Build history of the part. All positions in model axes, mm. A direction names the side the tool comes from. Round coordinates to 2 decimals unless told otherwise and drop trailing zeros. Write each loop counter-clockwise with the first axis right and the second up, starting at its lowest first coordinate (ties: lowest second). Pieces come first, ordered by that corner, then holes. Notation, with made-up numbers: M 3.25,59.5 L 32.25,59.5 A23 ccw 32.25,98.5 Z; hole C 50.5,-34 d6. An arc over 180 degrees is marked long. Write item = value, one per line.
from build123d import *

# Parameters (mm, degrees)
SKETCH1_W           = 60.96
SKETCH1_H           = 38.1
BOSS_EXTRUDE1_DEPTH = 104.775
SKETCH3_R           = 6.732897925
BOSS_EXTRUDE2_DEPTH = 20.0025
SKETCH2_R           = 6.865425502
BOSS_EXTRUDE3_DEPTH = 20.0025


with BuildPart() as part:
    # Sketch1 → Boss-Extrude1 (new body)
    with BuildSketch(Plane(origin=(0, 0, 0), x_dir=(0, 0, -1), z_dir=(1, 0, 0))):
        with Locations((30.48, 19.05)):
            Rectangle(SKETCH1_W, SKETCH1_H)
    extrude(amount=BOSS_EXTRUDE1_DEPTH)

    # Sketch3 → Boss-Extrude2 (add)
    with BuildSketch(Plane.ZY):
        with Locations((-46.280983346, 15.027703104)):
            Circle(SKETCH3_R)
    extrude(amount=BOSS_EXTRUDE2_DEPTH)

    # Sketch2 → Boss-Extrude3 (add)
    with BuildSketch(Plane(origin=(104.775, 0, 0), x_dir=(0, 0, -1), z_dir=(1, 0, 0))):
        with Locations(Location((14.493127779, 27.778848981, 0), (0, 0, 180))):
            Circle(SKETCH2_R)
    extrude(amount=BOSS_EXTRUDE3_DEPTH)


solid = part.part
1. Band-saw the part on D-D (z = -9). List the corners of the cut face in (x, y) (1 decimal), plus the area to 3 significant figures.
Responses:
outline = M 0,0 L 104.8,0 L 104.8,23.7 L 124.8,23.7 L 124.8,31.9 L 104.8,31.9 L 104.8,38.1 L 0,38.1 Z
area = 4,160 mm²
2. Band-saw the part on B-B (z = -56). List the corners of the cut face in (x, y) (3 decimals).
Responses:
outline = M 0,0 L 104.775,0 L 104.775,38.1 L 0,38.1 Z
3. Tool access for faces 1 (the face through (114.64, 34.48, -15.98)), 2 (the face through (-9.86, 17.05, -39.86)), 3 (the face through (52, 19, -60.96)): list every direction of +Z, -Z, +X, -X, +Y, -Y with a clear straight run to the whole face (end or side of a thin tool).
Responses:
face_1 = +X
face_2 = -X
face_3 = -Z, +X, -X, +Y, -Y
4. Flat gauge pins, fed straight in: pin 1 (5 mm diameter, centred on y = 30.5, z = -21, fed in from -X); pin 2 (6 mm diameter, centred on y = 25, z = -27.5, fed in from +X) (3 decimals). Where does each tip first touch, or does it go through?
Responses:
pin_1 = 0
pin_2 = 104.775
5. Band-saw the part on C-C (y = 3). List the corners of the cut face in (x, z) (3 decimals), plus the area to 3 significant figures.
Responses:
outline = M 0,-60.96 L 104.775,-60.96 L 104.775,0 L 0,0 Z
area = 6,390 mm²
6. Band-saw the part on A-A (y = 30). List the corners of the cut face in (x, z) (1 decimal), plus the area to 3 significant figures.
Responses:
outline = M 0,-61 L 104.8,-61 L 104.8,-21 L 124.8,-21 L 124.8,-8 L 104.8,-8 L 104.8,0 L 0,0 Z
area = 6,650 mm²
7. Probe probe 1 along X at (y, z) = (28.5, -49.5) (3 decimals); probe 2 along X at (y, z) = (12, -44) (1 decimal); probe 3 along Y at (x, z) = (-6, -51.5). List the from-to ranges inside material, lowest first.
Responses:
probe_1 = 0 to 104.775
probe_2 = -20 to 104.8
probe_3 = 10.77 to 19.28
